Could you check a few things on this model? Use its own coordinates, in mm. A direction names the side the tool comes from. Give positions to 0.01 mm unless a question says otherwise; leave off trailing zeros. Order: outer loops, then holes, each group sorted by start corner. A loop starts at its lowest first (then second) coordinate and runs counter-clockwise, first axis right, second up.
(1) If we mould it in two halves opening along Y, with no side actions, what happens to faces 5 (the flat face through (25, 130, -12)), 6 (the cylindrical face through (24.65, 131.88, -1.07)), 7 (the flat face through (25, 147, -23)), 8 (the cylindrical face through (23.591, 58.655, -1.479))? For each: released by +Y, released by -Y, zero draft, split by the parting line, or undercut.
(2) If I drill on probe 1 along Y at (x, z) = (38, -19.5); probe 2 along Z at (x, y) = (16, 67.5); probe 3 along Z at (x, y) = (44.5, -10), over which ranges is the centre line in solid material (lowest first)?
(3) Will these pins go through, and if not, where does the flat tip stop? pin 1 (12.5 mm diameter, centred on x = 30, z = -9.5, fed in from -Y); pin 2 (15 mm diameter, centred on x = 13.5, y = 96.5, fed in from -Z); pin 3 (5 mm diameter, centred on x = 16, z = -13.5, fed in from +Y).
(4) Imagine slicing it at B-B, the plane x = 25. Write out the boundary of the cut face in (y, z), then the cut area to 3 significant figures.
(5) On a 3-axis mill with a long thin cutter (end or side, diameter ignored), from which of +Z, -Z, +X, -X, +Y, -Y can I reach the whole of each face in a straight line? I mean faces 1 (the flat face through (0, 65, -2)), 2 (the flat face through (25, 147, -20)), 3 (the cylindrical face through (25.35, 131.07, -21.88)), 4 (the flat face through (25, -17, -20)). Say none if no direction works.
(6) Imagine slicing it at A-A, the plane z = -8.75. Write out the boundary of the cut face in (x, y), then the cut area to 3 significant figures.
(7) Imagine slicing it at C-C, the plane y = 65. Write out the boundary of the cut face in (x, z), then the cut area to 3 significant figures.
(8) Imagine slicing it at D-D, the plane x = 15. Write out the boundary of the cut face in (y, z), then the cut area to 3 significant figures.
from build123d import *

# Parameters (mm, degrees)
SKETCH_1_W                         = 50
SKETCH_1_H                         = 130
SM_BASE_FLANGE_1_DEPTH             = 3
SM_EDGE_FLANGE_1_STRIP_W           = 13.4732
SM_EDGE_FLANGE_1_STRIP_H           = 3
SM_EDGE_FLANGE_1_STRIP_CUT_DEPTH   = 50
SM_EDGE_FLANGE_1_STRIP_2_W         = 13.4732
SM_EDGE_FLANGE_1_STRIP_2_H         = 3
SM_EDGE_FLANGE_1_STRIP_CUT_2_DEPTH = 50
SM_EDGE_FLANGE_1_DEPTH             = 50
SM_EDGE_FLANGE_1_BEND_DEPTH        = 50
SM_EDGE_FLANGE_2_STRIP_W           = 13.4732
SM_EDGE_FLANGE_2_STRIP_H           = 3
SM_EDGE_FLANGE_2_STRIP_CUT_DEPTH   = 50
SM_EDGE_FLANGE_2_STRIP_2_W         = 13.4732
SM_EDGE_FLANGE_2_STRIP_2_H         = 3
SM_EDGE_FLANGE_2_STRIP_CUT_2_DEPTH = 50
SM_EDGE_FLANGE_2_DEPTH             = 50
SM_EDGE_FLANGE_2_BEND_DEPTH        = 50
SKETCH_18_R                        = 6.5
CUT_EXTRUDE_1_DEPTH                = 170.201063826


# Sheet-metal steps are written as plain solids
with BuildPart() as part:
    # Sketch 1 → 基体-法兰1 (new body)
    with BuildSketch(Plane.XY):
        with Locations((25, 65)):
            Rectangle(SKETCH_1_W, SKETCH_1_H)
    extrude(amount=-SM_BASE_FLANGE_1_DEPTH)

    # 边线-法兰1 strip (across the edge) → 边线-法兰1 strip cut (cut)
    with BuildSketch(Plane(origin=(0, 130, -3), x_dir=(0, -1, 0), z_dir=(1, 0, 0))):
        with Locations((-6, -1.5)):
            Rectangle(SM_EDGE_FLANGE_1_STRIP_W, SM_EDGE_FLANGE_1_STRIP_H)
    extrude(amount=SM_EDGE_FLANGE_1_STRIP_CUT_DEPTH, mode=Mode.SUBTRACT)

    # 边线-法兰1 strip 2 (across the edge) → 边线-法兰1 strip cut 2 (cut)
    with BuildSketch(Plane(origin=(50, 0, -3), x_dir=(0, 1, 0), z_dir=(-1, 0, 0))):
        with Locations((-6, -1.5)):
            Rectangle(SM_EDGE_FLANGE_1_STRIP_2_W, SM_EDGE_FLANGE_1_STRIP_2_H)
    extrude(amount=SM_EDGE_FLANGE_1_STRIP_CUT_2_DEPTH, mode=Mode.SUBTRACT)

    # 边线-法兰1 section (across the edge) → 边线-法兰1 (add)
    with BuildSketch(Plane(origin=(0, 130, -3), x_dir=(0, -1, 0), z_dir=(1, 0, 0))):
        with BuildLine():
            Line((-3, 0.7366), (-3, 17))
            Line((-3, 17), (0, 17))
            Line((0, 17), (0, 0.7366))
            ThreePointArc((0, 0.7366), (0.215745145, 0.215745145), (0.7366, 0))
            Line((0.7366, 0), (0.7366, -3))
            ThreePointArc((0.7366, -3), (-1.905575199, -1.905575199), (-3, 0.7366))
        make_face()
    extrude(amount=SM_EDGE_FLANGE_1_DEPTH)

    # 边线-法兰1 section 2 (across the edge) → 边线-法兰1 bend (add)
    with BuildSketch(Plane(origin=(50, 0, -3), x_dir=(0, 1, 0), z_dir=(-1, 0, 0))):
        with BuildLine():
            Line((-3, 0.7366), (-3, 17))
            Line((-3, 17), (0, 17))
            Line((0, 17), (0, 0.7366))
            ThreePointArc((0, 0.7366), (0.215745145, 0.215745145), (0.7366, 0))
            Line((0.7366, 0), (0.7366, -3))
            ThreePointArc((0.7366, -3), (-1.905575199, -1.905575199), (-3, 0.7366))
        make_face()
    extrude(amount=SM_EDGE_FLANGE_1_BEND_DEPTH)

    # 边线-法兰2 strip (across the edge) → 边线-法兰2 strip cut (cut)
    with BuildSketch(Plane(origin=(0, -3, -20), x_dir=(0, 0, 1), z_dir=(1, 0, 0))):
        with Locations((-6, -1.5)):
            Rectangle(SM_EDGE_FLANGE_2_STRIP_W, SM_EDGE_FLANGE_2_STRIP_H)
    extrude(amount=SM_EDGE_FLANGE_2_STRIP_CUT_DEPTH, mode=Mode.SUBTRACT)

    # 边线-法兰2 strip 2 (across the edge) → 边线-法兰2 strip cut 2 (cut)
    with BuildSketch(Plane(origin=(50, 133, -20), x_dir=(0, 0, 1), z_dir=(-1, 0, 0))):
        with Locations((-6, -1.5)):
            Rectangle(SM_EDGE_FLANGE_2_STRIP_2_W, SM_EDGE_FLANGE_2_STRIP_2_H)
    extrude(amount=SM_EDGE_FLANGE_2_STRIP_CUT_2_DEPTH, mode=Mode.SUBTRACT)

    # 边线-法兰2 section (across the edge) → 边线-法兰2 (add)
    with BuildSketch(Plane(origin=(0, -3, -20), x_dir=(0, 0, 1), z_dir=(1, 0, 0))):
        with BuildLine():
            Line((-3, 0.7366), (-3, 27))
            Line((-3, 27), (0, 27))
            Line((0, 27), (0, 0.7366))
            ThreePointArc((0, 0.7366), (0.215745145, 0.215745145), (0.7366, 0))
            Line((0.7366, 0), (0.7366, -3))
            ThreePointArc((0.7366, -3), (-1.905575199, -1.905575199), (-3, 0.7366))
        make_face()
    extrude(amount=SM_EDGE_FLANGE_2_DEPTH)

    # 边线-法兰2 section 2 (across the edge) → 边线-法兰2 bend (add)
    with BuildSketch(Plane(origin=(50, 133, -20), x_dir=(0, 0, 1), z_dir=(-1, 0, 0))):
        with BuildLine():
            Line((-3, 0.7366), (-3, 27))
            Line((-3, 27), (0, 27))
            Line((0, 27), (0, 0.7366))
            ThreePointArc((0, 0.7366), (0.215745145, 0.215745145), (0.7366, 0))
            Line((0.7366, 0), (0.7366, -3))
            ThreePointArc((0.7366, -3), (-1.905575199, -1.905575199), (-3, 0.7366))
        make_face()
    extrude(amount=SM_EDGE_FLANGE_2_BEND_DEPTH)

    # 草图18 → 切除-拉伸1 (cut, through all)
    with BuildSketch(Plane.XY):
        with Locations((25, 65)):
            Circle(SKETCH_18_R)
    extrude(amount=-CUT_EXTRUDE_1_DEPTH, mode=Mode.SUBTRACT)


solid = part.part
Answer block:
1. face 5: undercut
1. face 6: released by +Y
1. face 7: zero draft
1. face 8: undercut
2. probe 1: y = -3.04 to -0.01, 130.01 to 133.04
2. probe 2: z = -3 to 0
2. probe 3: z = -23 to -20
3. pin 1: stops at y = -3
3. pin 2: stops at z = -3
3. pin 3: stops at y = 133
4. outline: (-30, -23) - (-3.74, -23) arc R3.74 ccw to (0, -19.26) - (0, -3.74) arc R0.74 cw to (0.74, -3) - (58.5, -3) - (58.5, 0) - (0.74, 0) arc R3.74 ccw to (-3, -3.74) - (-3, -19.26) arc R0.74 cw to (-3.74, -20) - (-30, -20) - close; (71.5, -3) - (129.26, -3) arc R0.74 cw to (130, -3.74) - (130, -19.26) arc R3.74 ccw to (133.74, -23) - (160, -23) - (160, -20) - (133.74, -20) arc R0.74 cw to (133, -19.26) - (133, -3.74) arc R3.74 ccw to (129.26, 0) - (71.5, 0) - close
4. area: 639 mm2
5. face 1: +Z, -Z, -X, +Y, -Y
5. face 2: +Z, +X, -X, +Y
5. face 3: -Z, +X, -X
5. face 4: +Z, +X, -X, -Y
6. outline: (0, -3) - (50, -3) - (50, 0) - (0, 0) - close; (0, 130) - (50, 130) - (50, 133) - (0, 133) - close
6. area: 300 mm2
7. outline: (0, -3) - (18.5, -3) - (18.5, 0) - (0, 0) - close; (31.5, -3) - (50, -3) - (50, 0) - (31.5, 0) - close
7. area: 111 mm2
8. outline: (-30, -23) - (-3.74, -23) arc R3.74 ccw to (0, -19.26) - (0, -3.74) arc R0.74 cw to (0.74, -3) - (129.26, -3) arc R0.74 cw to (130, -3.74) - (130, -19.26) arc R3.74 ccw to (133.74, -23) - (160, -23) - (160, -20) - (133.74, -20) arc R0.74 cw to (133, -19.26) - (133, -3.74) arc R3.74 ccw to (129.26, 0) - (0.74, 0) arc R3.74 ccw to (-3, -3.74) - (-3, -19.26) arc R0.74 cw to (-3.74, -20) - (-30, -20) - close
8. area: 678 mm2
